Check sheet for the drawn part. Datum: minimum x, y, z corner. Units: mm. A direction names the side the tool comes from. Round coordinates to 2 decimals unless told otherwise and drop trailing zeros. Order: outer loops, then holes, each group sorted by start corner. A loop starts at its lowest first (then second) coordinate and runs counter-clockwise, first axis right, second up.
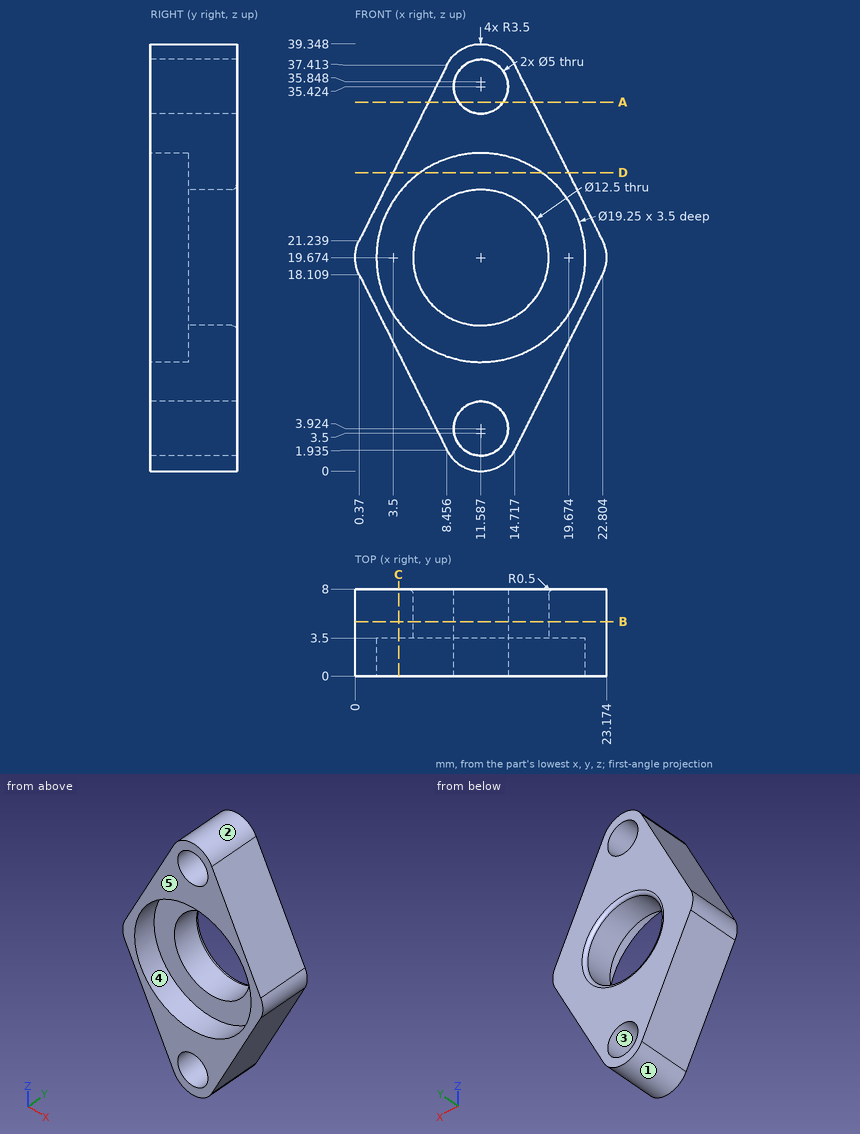
(1) Sectioned sample at A-A, the plane z = 34. Record the cut outline in (x, y).
Returned:
outline: (6.75, 0) - (9.53, 0) - (9.53, 8) - (6.75, 8) - close; (13.64, 0) - (16.42, 0) - (16.42, 8) - (13.64, 8) - close
(2) Draft check along Z on the marked faces 1, 2 and 3. Enter one of: released by +Z, released by -Z, zero draft, split by the parting line, or undercut.
Returned:
face 1: released by -Z
face 2: released by +Z
face 3: undercut
(3) Sectioned sample at C-C, the plane x = 4. Record the cut outline in (y, z).
Returned:
outline: (0, 10.85) - (8, 10.85) - (8, 28.5) - (0, 28.5) - (0, 25.6) - (3.5, 25.6) - (3.5, 13.75) - (0, 13.75) - close
(4) Set-up check for the marked faces 4 and 5: record each of +Z, -Z, +X, -X, +Y, -Y from which the full face is reachable in a straight line by a thin tool's end or side.
Returned:
face 4: -Y
face 5: +Z, -Z, +X, -X, -Y
(5) Material ranges on line 1 (X direction, y = 5, z = 19.5) (1 decimal); line 2 (Z direction, x = 10, y = 2.25) (1 decimal); line 3 (Y direction, x = 18, z = 16), recorded low to high.
Returned:
line 1: x = 0 to 5.3, 17.8 to 23.2
line 2: z = 0.4 to 2, 5.9 to 10.2, 29.2 to 33.5, 37.4 to 39
line 3: y = 3.5 to 8
(6) Depth check by flat-ended pin: P1, Ø4, axis at y = 7, z = 24, coming from the -X side; P2, Ø1.5, axis at y = 7, z = 32, coming from the -X side (1 decimal); P3, Ø6, axis at x = 7.5, z = 16.5, coming from the -Y side. Enter the tip coordinate at first touch or a pass-through.
Returned:
P1: stops at x = 0.75
P2: stops at x = 5.4
P3: stops at y = 3.5
(7) Sectioned sample at D-D, the plane z = 27.5. Record the cut outline in (x, y) (1 decimal).
Returned:
outline: (3.5, 0) - (6, 0) - (6, 3.5) - (17.2, 3.5) - (17.2, 0) - (19.7, 0) - (19.7, 8) - (3.5, 8) - close
(8) Sectioned sample at B-B, the plane y = 5. Give the number of separate pieces and of enclosed holes in the cut face, and give its area (3 significant figures).
Returned:
separate pieces: 1
enclosed holes: 3
area: 391 mm2
